```python
from build123d import *

# Parameters (mm, degrees)
BOSS_EXTRUDE1_DEPTH              = 665.1625
F_3_8_0_375_DIAMETER_HOLE1_D     = 9.525
F_3_8_0_375_DIAMETER_HOLE1_DEPTH = 11.684


with BuildPart() as part:
    # Sketch1 → Boss-Extrude1 (new body, symmetric)
    with BuildSketch(Plane(origin=(0, 0, 0), x_dir=(1, 0, 0), z_dir=(0, 1, 0))):
        with BuildLine():
            Line((-84.1375, 101.6), (84.1375, 101.6))
            Line((84.1375, 101.6), (84.1375, 89.916))
            Line((84.1375, 89.916), (10.31875, 89.916))
            ThreePointArc((10.31875, 89.916), (5.828621939, 88.056128061), (3.96875, 83.566))
            Line((3.96875, 83.566), (3.96875, -83.566))
            ThreePointArc((3.96875, -83.566), (5.828621939, -88.056128061), (10.31875, -89.916))
            Line((10.31875, -89.916), (84.1375, -89.916))
            Line((84.1375, -89.916), (84.1375, -101.6))
            Line((84.1375, -101.6), (-84.1375, -101.6))
            Line((-84.1375, -101.6), (-84.1375, -89.916))
            Line((-84.1375, -89.916), (-10.31875, -89.916))
            ThreePointArc((-10.31875, -89.916), (-5.828621939, -88.056128061), (-3.96875, -83.566))
            Line((-3.96875, -83.566), (-3.96875, 83.566))
            ThreePointArc((-3.96875, 83.566), (-5.828621939, 88.056128061), (-10.31875, 89.916))
            Line((-10.31875, 89.916), (-84.1375, 89.916))
            Line((-84.1375, 89.916), (-84.1375, 101.6))
        make_face()
    extrude(amount=BOSS_EXTRUDE1_DEPTH, both=True)

    # 3/8 (0.375) Diameter Hole1
    with Locations(Plane.XY.offset(101.6)):
        with Locations((-63.5, 255.5875), (63.5, 255.5875), (63.5, -455.6125), (63.5, -366.7125), (63.5, -277.8125), (63.5, -188.9125), (63.5, -100.0125), (63.5, -11.1125), (63.5, 77.7875), (-63.5, -455.6125), (-63.5, -366.7125), (-63.5, -277.8125), (-63.5, -188.9125), (-63.5, -100.0125), (-63.5, -11.1125), (-63.5, 77.7875), (-63.5, 166.6875), (63.5, 166.6875)):
            Hole(F_3_8_0_375_DIAMETER_HOLE1_D / 2, depth=F_3_8_0_375_DIAMETER_HOLE1_DEPTH)


solid = part.part
```
The model under review builds one solid part; all positions refer to its coordinate system, in mm. A direction names the side the tool comes from. Round coordinates to 2 decimals unless told otherwise and drop trailing zeros. Loops run counter-clockwise (first coordinate to the right, second up) from the corner with the lowest first, then second, coordinate; pieces in that order, holes last. Notation, with made-up numbers: (32, 28.25) - (62, 28.25) arc R14 ccw to (62, 41.25) - close; hole circle Ø8 at (-18.5, 80). An arc over 180 degrees is marked (long way). Write each question's results on one line, items separated by ' | '. Start each with the question number.
Q1. Tool access review of faces 1 (the flat face through (1, 9, 101.6)), 2 (the flat face through (47, 9, 89.916)), 3 (the flat face through (-47, 9, -89.916)): name each direction out of +Z, -Z, +X, -X, +Y, -Y from which nothing blocks a thin tool from reaching the whole face with its end or side.
Q2. Wall thickness on line 1 along Z through (x, y) = (-11, -474); line 2 along X through (y, z) = (331, 3); line 3 along X through (y, z) = (446, -88.5): over which ranges is each line inside the solid? List them lowest first. Write a range as [from, to].
Q3. Take a section at B-B on z = -33.5. Give the boundary of the cut face in (x, y), plus the area to 3 significant figures.
Q4. Insertion check: P1, Ø4, axis at y = -200.5, z = -49.5, coming from the +X side; P2, Ø7.5, axis at x = -63.5, y = -100.01, coming from the +Z side. Each pin has a flat end and moves straight along its axis. Give the tip position at first contact, or say it passes through.
Q5. Draft analysis for pull direction Z (two halves, no side actions). For faces 4 (the flat face through (3.969, 9, -1)), 5 (the flat face through (-1, 9, -101.6)), 6 (the flat face through (0, 665.162, -31)), state which applies: pulls with the +Z half, pulls with the -Z half, needs draft (parallel to the pull), parting line crosses it, or undercut.
Q6. Take a section at A-A on y = -75.5. Give the boundary of the cut face in (x, z), plus the area to 3 significant figures.
Data:
1) face 1: +Z, +X, -X, +Y, -Y | face 2: +X, +Y, -Y | face 3: -X, +Y, -Y
2) line 1: z = [-101.6, -89.92], [89.92, 101.6] | line 2: x = [-3.97, 3.97] | line 3: x = [-6.32, 6.32]
3) outline: (-3.97, -665.16) - (3.97, -665.16) - (3.97, 665.16) - (-3.97, 665.16) - close | area: 10,600 mm²
4) P1: stops at x = 3.97 | P2: stops at z = -89.92
5) face 4: undercut | face 5: pulls with the -Z half | face 6: needs draft
6) outline: (-84.14, -101.6) - (84.14, -101.6) - (84.14, -89.92) - (10.32, -89.92) arc R6.35 cw to (3.97, -83.57) - (3.97, 83.57) arc R6.35 cw to (10.32, 89.92) - (84.14, 89.92) - (84.14, 101.6) - (-84.14, 101.6) - (-84.14, 89.92) - (-10.32, 89.92) arc R6.35 cw to (-3.97, 83.57) - (-3.97, -83.57) arc R6.35 cw to (-10.32, -89.92) - (-84.14, -89.92) - close | area: 5,390 mm²
